Input: part model. Units: mm. Frame: model coordinates. Give positions to 0.01 mm unless a question says otherwise; leave off trailing zeros. Loops run counter-clockwise (first coordinate to the right, second up) from the corner with the lowest first, then second, coordinate; pieces in that order, holes last. Notation, with made-up numbers: (-5, 28) -> (39, 28) arc R21 ccw to (39, 66) -> close; hole circle Ø3 at (82, -10). An arc over 180 degrees is marked (long way). One line per question, with ' | ' between items.
from build123d import *

# Parameters (mm, degrees)
BOSS_EXTRUDE1_DEPTH = 4
SKETCH2_W           = 4
SKETCH2_H           = 27
CUT_EXTRUDE1_DEPTH  = 83.121860671
CUT_EXTRUDE2_DEPTH  = 83.121860671


with BuildPart() as part:
    # Sketch1 → Boss-Extrude1 (new body)
    with BuildSketch(Plane(origin=(0, 0, 0), x_dir=(1, 0, 0), z_dir=(0, 1, 0))):
        with BuildLine():
            Line((-58, 0), (58, 0))
            ThreePointArc((58, 0), (0, 58), (-58, 0))
        make_face()
    extrude(amount=BOSS_EXTRUDE1_DEPTH)

    # Sketch2 → Cut-Extrude1 (cut, through all)
    with BuildSketch(Plane(origin=(0, 4, 0), x_dir=(1, 0, 0), z_dir=(0, 1, 0))):
        with Locations((37, 13.5)):
            Rectangle(SKETCH2_W, SKETCH2_H)
        with Locations((-37, 13.5)):
            Rectangle(SKETCH2_W, SKETCH2_H)
    extrude(amount=-CUT_EXTRUDE1_DEPTH, mode=Mode.SUBTRACT)

    # Sketch3 → Cut-Extrude2 (cut, through all)
    with BuildSketch(Plane(origin=(0, 4, 0), x_dir=(1, 0, 0), z_dir=(0, 1, 0))):
        with BuildLine():
            Line((4, 38.663200531), (0, 38.663200531))
            Line((0, 38.663200531), (0, 0))
            Line((0, 0), (14, 0))
            ThreePointArc((14, 0), (12.017531054, 7.181848465), (6.631578947, 12.329726707))
            ThreePointArc((6.631578947, 12.329726707), (4.708024624, 14.16825465), (4, 16.733200531))
            Line((4, 16.733200531), (4, 38.663200531))
        make_face()
        with BuildLine():
            Line((-4, 38.663200531), (-4, 16.733200531))
            ThreePointArc((-4, 16.733200531), (-4.708024624, 14.16825465), (-6.631578947, 12.329726707))
            ThreePointArc((-6.631578947, 12.329726707), (-12.017531054, 7.181848465), (-14, 0))
            Line((-14, 0), (0, 0))
            Line((0, 0), (0, 38.663200531))
            Line((0, 38.663200531), (-4, 38.663200531))
        make_face()
    extrude(amount=-CUT_EXTRUDE2_DEPTH, mode=Mode.SUBTRACT)


solid = part.part
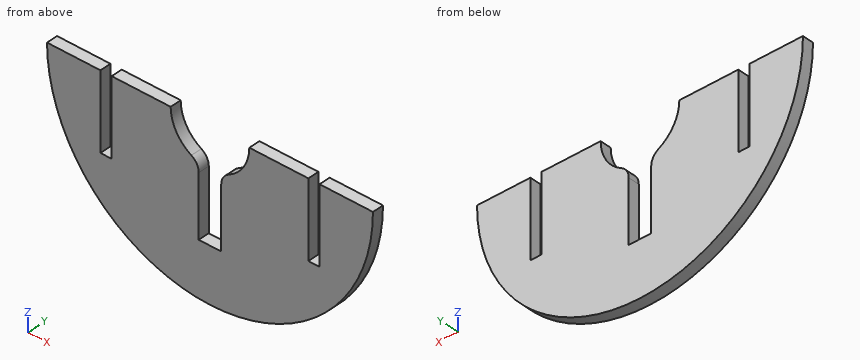
1. Section query D-D (x = 0). Output: boundary loops of the cut face in (y, z).
Determined:
outline: (0, -58) -> (4, -58) -> (4, -38.66) -> (0, -38.66) -> close
2. Ray query, line 1 along X through (y, z) = (1.6, -25.5); line 2 along X through (y, z) = (3.65, -1.5); line 3 along X through (y, z) = (3.1, -38). Return the intervals inside material, ascending. Write a range as from..to.
Determined:
line 1: x = -52.09..-39, -35..-4, 4..35, 39..52.09 | line 2: x = -57.98..-39, -35..-13.92, 13.92..35, 39..57.98 | line 3: x = -43.82..-4, 4..43.82
3. Section query B-B (z = -35). Output: boundary loops of the cut face in (x, y), then the cut area to 3 significant figures.
Determined:
outline: (-46.25, 0) -> (-4, 0) -> (-4, 4) -> (-46.25, 4) -> close; (4, 0) -> (46.25, 0) -> (46.25, 4) -> (4, 4) -> close | area: 338 mm2
4. Section query C-C (z = -9.5). Output: boundary loops of the cut face in (x, y), then the cut area to 3 significant figures.
Determined:
outline: (-57.22, 0) -> (-39, 0) -> (-39, 4) -> (-57.22, 4) -> close; (-35, 0) -> (-10.28, 0) -> (-10.28, 4) -> (-35, 4) -> close; (10.28, 0) -> (35, 0) -> (35, 4) -> (10.28, 4) -> close; (39, 0) -> (57.22, 0) -> (57.22, 4) -> (39, 4) -> close | area: 343 mm2
5. Pin query (flat end, axial travel): P1, Ø1.5, axis at x = 42.5, y = 1, coming from the -Z side; P2, Ø2, axis at y = 1.5, z = -15.5, coming from the +X side; P3, Ø4, axis at x = -35.5, z = -16, coming from the -Y side; P4, Ø2, axis at y = 2.5, z = -17.5, coming from the +X side. Return the tip coordinate at first contact, or that it passes through.
Determined:
P1: stops at z = -40.26 | P2: stops at x = 56.16 | P3: stops at y = 0 | P4: stops at x = 55.6
6. Section query A-A (y = 0.95). Output: boundary loops of the cut face in (x, z).
Determined:
outline: (-58, 0) arc R58 ccw to (58, 0) -> (39, 0) -> (39, -27) -> (35, -27) -> (35, 0) -> (14, 0) arc R14 cw to (6.63, -12.33) arc R5 ccw to (4, -16.73) -> (4, -38.66) -> (-4, -38.66) -> (-4, -16.73) arc R5 ccw to (-6.63, -12.33) arc R14 cw to (-14, 0) -> (-35, 0) -> (-35, -27) -> (-39, -27) -> (-39, 0) -> close
